Here's how the part is built. I have some questions about the finished solid (model axes, mm). A direction names the side the tool comes from. Coordinates: 2 decimals unless noted, no trailing zeros. Write each loop counter-clockwise with the first axis right and the second up, starting at its lowest first coordinate (ties: lowest second). Pieces come first, ordered by that corner, then holes.
Item 1: If we section it at B-B (y = 0): Please give me the cut outline in (x, z).
Item 2: If we section it at C-C (z = 38): Please give me the cut outline in (x, y), then the cut area to 3 significant figures.
Item 3: For faces 4 (the face through (8, 0, 12)), 5 (the face through (0, 14, 23)), 6 (the face through (-28, 0, -19)), which set-ups out of +Z, -Z, +X, -X, +Y, -Y let a thin tool reach every point of the face, with its end or its side?
Item 4: If we section it at A-A (z = 16.5): Please give me the cut outline in (x, y).
Item 5: I'm going to push flat-ended pins straight in: pin 1 Ø1 at (x, y) = (25, -12) entering from -Z; pin 2 Ø9.5 at (x, y) = (20, 0) entering from -Z; pin 3 Ø12 at (y, z) = (9.5, 25.5) entering from +X; pin 4 Ø20 at (x, y) = (-18.5, 6.5) entering from +Z. Where does each tip first touch, or does it pass through?
Item 6: If I drill on line 1 (Y direction, x = -19, z = 14); line 2 (Z direction, x = -20, y = 11.5); line 3 (Z direction, x = 13, y = 4.5), over which ranges is the centre line in solid material (lowest first)?
Item 7: If we section it at D-D (y = 16): Please give me the cut outline in (x, z).
Item 8: We'd pull the mould along X, two halves only. Please class faces 1 (the face through (12, 0, 6)), 2 (the face through (-40, 0, -9)), 3 (the face through (40, 0, 6)): +X half, -X half, draft (parallel to the pull), parting line (faces both ways), or undercut.
Solid Edge part; units mm, degrees
sketch "Sketch1" plane through (0, 0, 0) normal (0, 0, 1) x (1, 0, 0)
  line L0 (-40, -20) -> (20, -20)
  line L1 (-40, 20) -> (-40, -20)
  line L2 (8, 20) -> (-40, 20)
  line L3 (20, 20) -> (8, 20)
  arc A0 (20, 20) -> (20, -20) centre (20, 0) cw
  circle A1 centre (20, 0) radius 8
extrude "ExtrudedProtrusion_1" add sketch "Sketch1" along normal blind 12
sketch "Sketch2" plane through (0, -20, 0) normal (0, -1, 0) x (1, 0, 0)
  line L0 (0, 32) -> (0, 12)
  line L1 (0, 12) -> (-40, 12)
  line L2 (-40, 12) -> (-40, 32)
  arc A0 (-40, 32) -> (0, 32) centre (-20, 32) cw
  circle A1 centre (-20, 32) radius 8
extrude "ExtrudedProtrusion_2" add sketch "Sketch2" against normal blind 12
mirror "Mirror1" about plane through (0, 0, 0) normal (0, -1, 0) of "ExtrudedProtrusion_2"
sketch "Sketch3" plane through (-40, 0, 0) normal (1, 0, 0) x (0, 1, 0)
  line L0 (-20, 0) -> (-20, -28)
  line L1 (20, -28) -> (20, 0)
  line L2 (20, 0) -> (-20, 0)
  arc A0 (20, -28) -> (-20, -28) centre (0, -28) cw
  circle A1 centre (0, -28) radius 8
extrude "ExtrudedProtrusion_4" add sketch "Sketch3" along normal blind 12
fillet "Round_2" radius 2 1 edges at (0, -14, 12)
fillet "Round_3" radius 2 1 edges at (0, 14, 12)
Answer list:
1. outline: (-40, -48) - (-28, -48) - (-28, -36) - (-40, -36) - close; (-40, -20) - (-28, -20) - (-28, 0) - (12, 0) - (12, 12) - (-40, 12) - close; (28, 0) - (40, 0) - (40, 12) - (28, 12) - close
2. outline: (-39.08, -20) - (-25.29, -20) - (-25.29, -8) - (-39.08, -8) - close; (-39.08, 8) - (-25.29, 8) - (-25.29, 20) - (-39.08, 20) - close; (-14.71, -20) - (-0.92, -20) - (-0.92, -8) - (-14.71, -8) - close; (-14.71, 8) - (-0.92, 8) - (-0.92, 20) - (-14.71, 20) - close
2. area: 662 mm2
3. face 4: +Z, +X
3. face 5: +Z, +X, +Y, -Y
3. face 6: -Z, +X, +Y, -Y
4. outline: (-40, -20) - (0, -20) - (0, -8) - (-40, -8) - close; (-40, 8) - (0, 8) - (0, 20) - (-40, 20) - close
5. pin 1: stops at z = 0
5. pin 2: passes through
5. pin 3: stops at x = 0
5. pin 4: stops at z = 52
6. line 1: y = -20 to -8, 8 to 20
6. line 2: z = 0 to 24, 40 to 52
6. line 3: z = 0 to 12
7. outline: (-40, -40) - (-28, -40) - (-28, 0) - (32, 0) - (32, 12) - (2, 12) arc R2 cw to (0, 14) - (0, 32) arc R20 ccw to (-40, 32) - close; hole circle Ø16 at (-20, 32)
8. face 1: undercut
8. face 2: -X half
8. face 3: +X half
